```python
from build123d import *

# Parameters (mm, degrees)
F0_R         = 2.6
F1_DEPTH     = 2
F2_R         = 2.25
F3_DEPTH     = 8
F4_R         = 2.6
F5_DEPTH     = 2
F8_DEPTH     = 5
F10_DEPTH    = 5
F11_C1_SIZE2 = 1
F11_C1_SIZE  = 1.7320508076
F11_C2_SIZE2 = 1
F11_C2_SIZE  = 1.7320508076
F12_C1_SIZE2 = 1
F12_C1_SIZE  = 1.7320508076
F12_C2_SIZE2 = 1
F12_C2_SIZE  = 1.7320508076
F13_R        = 0.5
F15_DEPTH    = 25


# Not quite as in the source:
# - a fillet or chamfer that OpenCascade refuses, or shapes differently, is made with other operations: its cross-section is extruded or revolved along the edge and cut away or added


with BuildPart() as f1:
    # F0 (on Top) → F1 (new body)
    with BuildSketch(Plane.XY):
        Circle(F0_R)
    extrude(amount=F1_DEPTH)

    # F2 (on face) → F3 (join)
    with BuildSketch(Plane.XY.offset(2)):
        Circle(F2_R)
    extrude(amount=F3_DEPTH)

    # F4 (on face) → F5 (join)
    with BuildSketch(Plane.XY.offset(10)):
        Circle(F4_R)
    extrude(amount=F5_DEPTH)

    # F6: fillet of radius 0.5 on 2 edges, made by hand

    # F6_s1 → F6_t2 (revolve, cut)
    with BuildSketch(Plane.XZ):
        with BuildLine():
            ThreePointArc((2.25, 2), (2.5031128874, 1.8188343884), (2.6, 1.5230303993))
            Line((2.6, 1.5230303993), (2.6, 2))
            Line((2.6, 2), (2.25, 2))
        make_face()
    revolve(axis=Axis((0, 0, 2), (0, 0, 1)), mode=Mode.SUBTRACT)

    # F6_s3 → F6_t4 (revolve, cut)
    with BuildSketch(Plane.XZ):
        with BuildLine():
            ThreePointArc((2.6, 10.4769696007), (2.5031128874, 10.1811656116), (2.25, 10))
            Line((2.25, 10), (2.6, 10))
            Line((2.6, 10), (2.6, 10.4769696007))
        make_face()
    revolve(axis=Axis((0, 0, 10), (0, 0, 1)), mode=Mode.SUBTRACT)

    # F7 (on face) → F8 (cut)
    with BuildSketch(Plane(origin=(0, 0, 0), x_dir=(1, 0, 0), z_dir=(0, 0, -1))):
        with BuildLine():
            ThreePointArc((-2.4894778569, 0.75), (-2.6, 0), (-2.4894778569, -0.75))
            Line((-2.4894778569, -0.75), (2.4894778569, -0.75))
            ThreePointArc((2.4894778569, -0.75), (2.6, 0), (2.4894778569, 0.75))
            Line((2.4894778569, 0.75), (-2.4894778569, 0.75))
        make_face()
    extrude(amount=-F8_DEPTH, mode=Mode.SUBTRACT)

    # F9 (on face) → F10 (cut)
    with BuildSketch(Plane.XY.offset(12)):
        with BuildLine():
            ThreePointArc((-2.4894778569, 0.75), (-2.6, 0), (-2.4894778569, -0.75))
            Line((-2.4894778569, -0.75), (2.4894778569, -0.75))
            ThreePointArc((2.4894778569, -0.75), (2.6, 0), (2.4894778569, 0.75))
            Line((2.4894778569, 0.75), (-2.4894778569, 0.75))
        make_face()
    extrude(amount=-F10_DEPTH, mode=Mode.SUBTRACT)

    # F11: chamfer of 1 x 1.7320508076 on 2 edges, made by hand

    # F11_c1
    f11_c1_edges = [f1.edges().sort_by_distance(p)[0] for p in [
        (0, 2.6, 0),
    ]]
    f11_c1_side = f1.faces().sort_by_distance((0, 2.58, 0))[0]
    chamfer(f11_c1_edges, length=F11_C1_SIZE, length2=F11_C1_SIZE2, reference=f11_c1_side)

    # F11_c2
    f11_c2_edges = [f1.edges().sort_by_distance(p)[0] for p in [
        (0, -2.6, 0),
    ]]
    f11_c2_side = f1.faces().sort_by_distance((0, -2.58, 0))[0]
    chamfer(f11_c2_edges, length=F11_C2_SIZE, length2=F11_C2_SIZE2, reference=f11_c2_side)

    # F12: chamfer of 1 x 1.7320508076 on 2 edges, made by hand

    # F12_c1
    f12_c1_edges = [f1.edges().sort_by_distance(p)[0] for p in [
        (0, -2.6, 12),
    ]]
    f12_c1_side = f1.faces().sort_by_distance((0, -2.58, 12))[0]
    chamfer(f12_c1_edges, length=F12_C1_SIZE, length2=F12_C1_SIZE2, reference=f12_c1_side)

    # F12_c2
    f12_c2_edges = [f1.edges().sort_by_distance(p)[0] for p in [
        (0, 2.6, 12),
    ]]
    f12_c2_side = f1.faces().sort_by_distance((0, 2.58, 12))[0]
    chamfer(f12_c2_edges, length=F12_C2_SIZE, length2=F12_C2_SIZE2, reference=f12_c2_side)

    # F13
    f13_edges = [f1.edges().sort_by_distance(p)[0] for p in [
        (0, -2.6, 11),
        (0, 2.6, 11),
        (0, -2.6, 1),
        (0, 2.6, 1),
    ]]
    fillet(f13_edges, radius=F13_R)

    # F14 (on face) → F15 (cut)
    with BuildSketch(Plane.XY.offset(12)):
        with BuildLine():
            Line((-1.85, -1.8268825906), (-1.85, 1.8268825906))
            ThreePointArc((-1.85, 1.8268825906), (-2.6, 0), (-1.85, -1.8268825906))
        make_face()
    extrude(amount=-F15_DEPTH, mode=Mode.SUBTRACT)


solid = f1.part
```
The model under review builds one solid part; all positions refer to its coordinate system, in mm. A direction names the side the tool comes from. Round coordinates to 2 decimals unless told otherwise and drop trailing zeros. Order: outer loops, then holes, each group sorted by start corner. A loop starts at its lowest first (then second) coordinate and runs counter-clockwise, first axis right, second up. Notation, with made-up numbers: (59, -12.5) - (114, -12.5) arc R13 cw to (114, -3.5) - close; hole circle Ø9 at (78, -10.75). An arc over 180 degrees is marked (long way). Answer in a Markdown table with one row per item.
(1) Clearance check with flat-ended pins moving along their axes: P1, Ø1.3, axis at x = -0.5, z = 2.5, coming from the -Y side; P2, Ø1.2, axis at x = -0.5, y = 0, coming from the -Z side; P3, Ø3, axis at y = 1.5, z = 5.5, coming from the +X side. State where each tip first meets the part, or that it passes through.
Result set:
| item | result |
|---|---|
| P1 | stops at y = -2.44 |
| P2 | stops at z = 5 |
| P3 | stops at x = 2.25 |
(2) Take a section at B-B on y = 0. Write out the cut boundary in (x, z), plus the area to 3 significant figures.
Result set:
| item | result |
|---|---|
| outline | (-1.85, 5) - (2.25, 5) - (2.25, 7) - (-1.85, 7) - close |
| area | 8.20 mm2 |
(3) Take a section at A-A on z = 8.5. Write out the cut boundary in (x, y), plus the area to 3 significant figures.
Result set:
| item | result |
|---|---|
| outline | (-1.85, -1.28) arc R2.25 ccw to (2.12, -0.75) - (-1.85, -0.75) - close; (-1.85, 0.75) - (2.12, 0.75) arc R2.25 ccw to (-1.85, 1.28) - close |
| area | 9.12 mm2 |
(4) Take a section at C-C on z = 6.5. Write out the cut boundary in (x, y), plus the area to 3 significant figures.
Result set:
| item | result |
|---|---|
| outline | (-1.85, -1.28) arc R2.25 ccw (long way) to (-1.85, 1.28) - close |
| area | 15.2 mm2 |
(5) For line 1 (Y direction, x = -0.4, z = 7.25); line 2 (Y direction, x = 1.8, z = 2.5); line 3 (Z direction, x = 0.5, y = -2.3), list the stretches that pass through material, from the lowest coordinate up. Write a range as from..to.
Result set:
| item | result |
|---|---|
| line 1 | y = -2.21..-0.75, 0.75..2.21 |
| line 2 | y = -1.35..-0.75, 0.75..1.35 |
| line 3 | z = 0.86..1.95, 10.05..11.14 |
(6) Mouldability with a two-part tool opening along Z and no side actions: class faces 1 (the face through (2.25, -0.08, 5.94)), 2 (the face through (0, 0, 7)), 3 (the face through (0, -0.75, 10)) as released by +Z, released by -Z, zero draft, split by the parting line, or undercut.
Result set:
| item | result |
|---|---|
| face 1 | undercut |
| face 2 | released by +Z |
| face 3 | zero draft |
(7) Take a section at D-D on z = 1.75. Write out the cut boundary in (x, y).
Result set:
| item | result |
|---|---|
| outline | (-1.85, -1.75) arc R2.55 ccw to (2.43, -0.75) - (-1.85, -0.75) - close; (-1.85, 0.75) - (2.43, 0.75) arc R2.55 ccw to (-1.85, 1.75) - close |
(8) Machinability: for faces 4 (the face through (0.019, -1.455, 0.339)), 5 (the face through (0, 0.75, 10)), 6 (the face through (0, -0.75, 2)), which of the approach directions +Z, -Z, +X, -X, +Y, -Y give a long, thin tool a straight path to every point of the face, cutting with its end or side? Answer none if there is none.
Result set:
| item | result |
|---|---|
| face 4 | -Z, -Y |
| face 5 | +Z, +X, -X |
| face 6 | -Z, +X, -X |
